```python
from build123d import *

# Parameters (mm, degrees)
SKETCH_1_R               = 20
EXTRUDE_1_DEPTH          = 5
CUT_EXTRUDE_1_REACH      = 87.2
SKETCH_2_R               = 3
MIRROR_2_COPY_1_REACH    = 87.2
MIRROR_2_COPY_1_SKETCH_R = 3
SKETCH_3_R               = 1.5
CUT_EXTRUDE_2_DEPTH      = 86.199993462
PATTERN_CIRCULAR_1_COUNT = 6


with BuildPart() as part:
    # 草图1 → 凸台-拉伸1 (new body)
    with BuildSketch(Plane(origin=(0, 0, 0), x_dir=(1, 0, 0), z_dir=(0, 1, 0))):
        with BuildLine():
            Line((46.623322285, 16.328680875), (65.781966365, 25.910071498))
            ThreePointArc((65.781966365, 25.910071498), (68.576327064, 34.295567803), (60.190830759, 37.089928502))
            Line((60.190830759, 37.089928502), (41.03218668, 27.50853788))
            ThreePointArc((41.03218668, 27.50853788), (0, 49.4), (-41.03218668, 27.50853788))
            Line((-41.03218668, 27.50853788), (-60.190830759, 37.089928502))
            ThreePointArc((-60.190830759, 37.089928502), (-68.576327064, 34.295567803), (-65.781966365, 25.910071498))
            Line((-65.781966365, 25.910071498), (-46.623322285, 16.328680875))
            ThreePointArc((-46.623322285, 16.328680875), (-49.4, 0), (-46.623322285, -16.328680875))
            Line((-46.623322285, -16.328680875), (-65.781966365, -25.910071498))
            ThreePointArc((-65.781966365, -25.910071498), (-68.576327064, -34.295567803), (-60.190830759, -37.089928502))
            Line((-60.190830759, -37.089928502), (-41.03218668, -27.50853788))
            ThreePointArc((-41.03218668, -27.50853788), (0, -49.4), (41.03218668, -27.50853788))
            Line((41.03218668, -27.50853788), (60.190830759, -37.089928502))
            ThreePointArc((60.190830759, -37.089928502), (68.576327064, -34.295567803), (65.781966365, -25.910071498))
            Line((65.781966365, -25.910071498), (46.623322285, -16.328680875))
            ThreePointArc((46.623322285, -16.328680875), (49.4, 0), (46.623322285, 16.328680875))
        make_face()
        with Locations(Location((0, 0, 0), (0, 0, 270))):
            Circle(SKETCH_1_R, mode=Mode.SUBTRACT)
    extrude(amount=EXTRUDE_1_DEPTH)

    # 草图2 → 切除-拉伸1 (cut, up to next)
    with BuildSketch(Plane(origin=(0, 5, 0), x_dir=(1, 0, 0), z_dir=(0, 1, 0)), mode=Mode.PRIVATE) as cut_extrude_1_sk1:
        with Locations(Location((-62.986398562, 31.5, 0), (0, 0, 270))):
            Circle(SKETCH_2_R)
    cut_extrude_1_tool1 = extrude(cut_extrude_1_sk1.sketch, amount=-CUT_EXTRUDE_1_REACH, mode=Mode.PRIVATE) & part.part
    cut_extrude_1 = cut_extrude_1_tool1.solids().sort_by_distance((-62.986399, 5, -31.5))[0]
    add(cut_extrude_1, mode=Mode.SUBTRACT)

    # 镜向1: 切除-拉伸1 across plane
    add(cut_extrude_1.mirror(Plane.XY), mode=Mode.SUBTRACT)

    # 镜向2: 切除-拉伸1 across plane
    add(cut_extrude_1.mirror(Plane(origin=(0, 0, 0), x_dir=(0, 0, 1), z_dir=(1, 0, 0))), mode=Mode.SUBTRACT)

    # 镜向2 copy 1 sketch → 镜向2 copy 1 (cut, up to next)
    with BuildSketch(Plane(origin=(0, 5, 0), x_dir=(-1, 0, 0), z_dir=(0, 1, 0)), mode=Mode.PRIVATE) as mirror_2_copy_1_sk1:
        with Locations(Location((-62.986398562, 31.5, 0), (0, 0, 270))):
            Circle(MIRROR_2_COPY_1_SKETCH_R)
    mirror_2_copy_1_tool1 = extrude(mirror_2_copy_1_sk1.sketch, amount=-MIRROR_2_COPY_1_REACH, mode=Mode.PRIVATE) & part.part
    add(mirror_2_copy_1_tool1.solids().sort_by_distance((62.986399, 5, 31.5))[0], mode=Mode.SUBTRACT)

    # 草图3 → 切除-拉伸2 (cut, through all)
    with BuildSketch(Plane.XZ):
        with Locations(Location((0, 43.5, 0), (0, 0, 270))):
            Circle(SKETCH_3_R)
    cut_extrude_2 = extrude(amount=-CUT_EXTRUDE_2_DEPTH, mode=Mode.SUBTRACT)

    # 阵列(圆周)1: 切除-拉伸2 ×6 about axis
    pattern_circular_1_axis = Axis((0, 0, 0), (0, 1, 0))
    for i in range(1, PATTERN_CIRCULAR_1_COUNT):
        add(cut_extrude_2.rotate(pattern_circular_1_axis, i * 360 / PATTERN_CIRCULAR_1_COUNT), mode=Mode.SUBTRACT)


solid = part.part
```
Verification items for the finished model (mm, model axes). A direction names the side the tool comes from. Give positions to 0.01 mm unless a question says otherwise; leave off trailing zeros. Write each loop counter-clockwise with the first axis right and the second up, starting at its lowest first coordinate (ties: lowest second). Pieces come first, ordered by that corner, then holes. Notation, with made-up numbers: (29.5, -5) - (82.5, -5) arc R27 ccw to (82.5, 16) - close; hole circle Ø1 at (72, 55.25). An arc over 180 degrees is marked (long way). Put each result on its own line as item: value.
Q1. Section check A-A on z = 0. Record the cut outline in (x, y), and give its area (3 significant figures).
Result:
outline: (-49.4, 0) - (-20, 0) - (-20, 5) - (-49.4, 5) - close; (20, 0) - (49.4, 0) - (49.4, 5) - (20, 5) - close
area: 294 mm2
Q2. Depth check by flat-ended pin: P1, Ø3, axis at x = 36, y = 3.5, coming from the +Z side. Enter the tip coordinate at first touch or a pass-through.
Result:
P1: z = 35.36
Q3. Section check C-C on y = 2.85. Count the separate pieces of the cut face and the enclosed holes in it, and give its area (3 significant figures).
Result:
separate pieces: 1
enclosed holes: 11
area: 7,560 mm2
Q4. Section check D-D on z = 31. Record the cut outline in (x, y), and give its area (3 significant figures).
Result:
outline: (-69.22, 0) - (-65.94, 0) - (-65.94, 5) - (-69.22, 5) - close; (-60.03, 0) - (-48.01, 0) - (-48.01, 5) - (-60.03, 5) - close; (-38.46, 0) - (38.46, 0) - (38.46, 5) - (-38.46, 5) - close; (48.01, 0) - (60.03, 0) - (60.03, 5) - (48.01, 5) - close; (65.94, 0) - (69.22, 0) - (69.22, 5) - (65.94, 5) - close
area: 537 mm2
Q5. Section check B-B on x = 0. Record the cut outline in (y, z), and give its area (3 significant figures).
Result:
outline: (0, -49.4) - (5, -49.4) - (5, -45) - (0, -45) - close; (0, -42) - (5, -42) - (5, -20) - (0, -20) - close; (0, 20) - (5, 20) - (5, 42) - (0, 42) - close; (0, 45) - (5, 45) - (5, 49.4) - (0, 49.4) - close
area: 264 mm2
Q6. Scan lines: probe 1 along Z at (x, y) = (37, 0.8); probe 2 along X at (y, z) = (1.4, -31.5); probe 3 along X at (y, z) = (3, 0). Record each from-to range of solid material in increasing order. Write a range as from..to.
Result:
probe 1: -32.73..-23.09, -20.41..20.41, 23.09..32.73
probe 2: -69.24..-65.99, -59.99..-49.01, -38.05..38.05, 49.01..59.99, 65.99..69.24
probe 3: -49.4..-20, 20..49.4
Q7. Set-up check for faces 1 (the face through (56.34, 2.46, 21.19)), 2 (the face through (-56.069, 2.465, 21.052)), 3 (the face through (50.477, 2.465, 32.232)), 4 (the face through (-50.477, 2.465, -32.232)): record each of +Z, -Z, +X, -X, +Y, -Y from which the full face is reachable in a straight line by a thin tool's end or side.
Result:
face 1: +X, +Y, -Y
face 2: -X, +Y, -Y
face 3: +Z, +Y, -Y
face 4: -Z, +Y, -Y
